The model under review builds one solid part; all positions refer to its coordinate system, in mm. A direction names the side the tool comes from. Give positions to 0.01 mm unless a question says otherwise; leave off trailing zeros. Loops run counter-clockwise (first coordinate to the right, second up) from the corner with the lowest first, then second, coordinate; pieces in that order, holes last. Notation, with made-up numbers: M 47,40.5 L 100,40.5 A18 cw 100,52.5 Z; hole C 44,73.25 d2. An arc over 180 degrees is marked long. Write item = value, one per line. Start each with the question number.
1. We need section C-C on x = 6. Give the boundary of the cut face in (y, z).
2. For faces 1 (the face through (9.282, 0, 5)), 2 (the face through (-36, 9.552, 5)), 3 (the face through (-11, -10, 6)), 4 (the face through (12.282, 1, 5)), list the 3-axis set-ups (+Z, -Z, +X, -X, +Y, -Y) from which the entire face can be reached by the end or side of a thin tool; tool diameter is ignored.
3. For pin 1 (4 mm diameter, centred on x = 2, z = 5, fed in from -Y); pin 2 (10 mm diameter, centred on x = -3.5, y = -7, fed in from -Z); pin 3 (3 mm diameter, centred on y = 2, z = 6, fed in from +X), all flat-tipped, find the tip position at first contact; note any pin that passes through.
4. Draft analysis for pull direction Z (two halves, no side actions). For faces 5 (the face through (10.76, -2.55, 4.24)), 6 (the face through (-12, -8.238, 8)), 7 (the face through (-11, 11, 6)), state which applies: pulls with the +Z half, pulls with the -Z half, needs draft (parallel to the pull), parting line crosses it, or undercut.
5. Wall thickness on line 1 along Y through (x, z) = (-33.8, 5); line 2 along X through (y, z) = (0, 2.5); line 3 along X through (y, z) = (10, 0.5): over which ranges is each line inside the solid? List them lowest first. Write a range as from..to.
6. We need section D-D on z = 9. Give the boundary of the cut face in (x, y), then the cut area to 3 significant figures.
7. We need section B-B on z = 3.5. Give the boundary of the cut face in (x, y), then the cut area to 3 significant figures.
8. We need section A-A on y = -0.75. Give the boundary of the cut face in (x, z).
from build123d import *

# Parameters (mm, degrees)
SKETCH1_W                    = 41
SKETCH1_H                    = 17.79
BOSS_EXTRUDE1_DEPTH          = 10
M2_5X0_45_TAPPED_HOLE2_D     = 2.05
M2_5X0_45_TAPPED_HOLE2_DEPTH = 7.25
M2_5X0_45_TAPPED_HOLE2_TIP   = 0.615882135
M2_5X0_45_TAPPED_HOLE1_D     = 2.05
M2_5X0_45_TAPPED_HOLE1_DEPTH = 7.25
M2_5X0_45_TAPPED_HOLE1_TIP   = 0.615882135
SKETCH10_W                   = 41
SKETCH10_H                   = 3
CUT_EXTRUDE1_DEPTH           = 6


with BuildPart() as part:
    # Sketch1 → Boss-Extrude1 (new body)
    with BuildSketch(Plane.XY):
        Polygon((12.281684518, 9.551958914), (15.281684518, 9.551958914), (15.281684518, 12.551958914), (-37.718315482, 12.551958914), (-37.718315482, 9.551958914), (-34.718315482, 9.551958914), (-34.718315482, -8.238041086), (-37.718315482, -8.238041086), (-37.718315482, -11.238041086), (15.281684518, -11.238041086), (15.281684518, -8.238041086), (12.281684518, -8.238041086), align=None)
        with Locations((-11.218315482, 0.656958914)):
            Rectangle(SKETCH1_W, SKETCH1_H, mode=Mode.SUBTRACT)
    extrude(amount=BOSS_EXTRUDE1_DEPTH)

    # M2.5x0.45 Tapped Hole2
    with Locations(Plane.ZY.offset(34.718315482)):
        with Locations((5, 4.551958914), (5, -3.238041086)):
            Hole(M2_5X0_45_TAPPED_HOLE2_D / 2, depth=M2_5X0_45_TAPPED_HOLE2_DEPTH)
            with Locations((0, 0, -(M2_5X0_45_TAPPED_HOLE2_DEPTH + M2_5X0_45_TAPPED_HOLE2_TIP / 2))):  # 118° drill point
                Cone(0, M2_5X0_45_TAPPED_HOLE2_D / 2, M2_5X0_45_TAPPED_HOLE2_TIP, mode=Mode.SUBTRACT)

    # M2.5x0.45 Tapped Hole1
    with Locations(Plane(origin=(12.281684518, 2.476678441, 1.606875776), x_dir=(0, 0, -1), z_dir=(1, 0, 0))):
        with Locations((-3.393124224, 2.075280473), (-3.393124224, -5.714719527)):
            Hole(M2_5X0_45_TAPPED_HOLE1_D / 2, depth=M2_5X0_45_TAPPED_HOLE1_DEPTH)
            with Locations((0, 0, -(M2_5X0_45_TAPPED_HOLE1_DEPTH + M2_5X0_45_TAPPED_HOLE1_TIP / 2))):  # 118° drill point
                Cone(0, M2_5X0_45_TAPPED_HOLE1_D / 2, M2_5X0_45_TAPPED_HOLE1_TIP, mode=Mode.SUBTRACT)

    # Sketch10 → Cut-Extrude1 (cut)
    with BuildSketch(Plane(origin=(0, 0, 0), x_dir=(-1, 0, 0), z_dir=(0, 0, -1))):
        with Locations((11.218315482, -9.738041086)):
            Rectangle(SKETCH10_W, SKETCH10_H)
    cut_extrude1 = extrude(amount=-CUT_EXTRUDE1_DEPTH, mode=Mode.SUBTRACT)

    # Mirror3: Cut-Extrude1 across plane
    add(cut_extrude1.mirror(Plane.ZX.offset(0.656958914)), mode=Mode.SUBTRACT)


solid = part.part
Final values:
q1.outline = M -11.24,6 L -8.24,6 L -8.24,10 L -11.24,10 Z; M 9.55,6 L 12.55,6 L 12.55,10 L 9.55,10 Z
q2.face_1 = -Z
q2.face_2 = +Z, -Z, -X
q2.face_3 = -Z, +Y, -Y
q2.face_4 = +Z, -Z, +X
q3.pin_1 = -11.24
q3.pin_2 = 6
q3.pin_3 = 12.28
q4.face_5 = undercut
q4.face_6 = needs draft
q4.face_7 = pulls with the -Z half
q5.line_1 = -11.24..-4.26, -2.21..3.53, 5.58..12.55
q5.line_2 = -34.72..-31.72, 9.28..12.28
q5.line_3 = -37.72..-31.72, 9.28..15.28
q6.outline = M -37.72,-11.24 L 15.28,-11.24 L 15.28,-8.24 L 12.28,-8.24 L 12.28,9.55 L 15.28,9.55 L 15.28,12.55 L -37.72,12.55 L -37.72,9.55 L -34.72,9.55 L -34.72,-8.24 L -37.72,-8.24 Z; hole M -31.72,-8.24 L 9.28,-8.24 L 9.28,9.55 L -31.72,9.55 Z
q6.area = 425 mm²
q7.outline = M -37.72,-11.24 L -31.72,-11.24 L -31.72,12.55 L -37.72,12.55 L -37.72,9.55 L -34.72,9.55 L -34.72,-8.24 L -37.72,-8.24 Z; M 9.28,-11.24 L 15.28,-11.24 L 15.28,-8.24 L 12.28,-8.24 L 12.28,9.55 L 15.28,9.55 L 15.28,12.55 L 9.28,12.55 Z
q7.area = 179 mm²
q8.outline = M -34.72,0 L -31.72,0 L -31.72,10 L -34.72,10 Z; M 9.28,0 L 12.28,0 L 12.28,10 L 9.28,10 Z
